Source: CAD feature listing. Evaluate the final solid. Frame: model axes, mm. A direction names the side the tool comes from. Give positions to 0.01 mm unless a question says otherwise; leave off trailing zeros. Order: outer loops, then holes, each group sorted by start corner. A loop starts at its lowest first (then second) coordinate and runs counter-clockwise, first axis right, second up. Notation, with made-up numbers: (77, 37.25) - (126, 37.25) arc R18 ccw to (126, 58.25) - close; hole circle Ø4 at (21.5, 79.25). An arc over 180 degrees is marked (long way). One line per item, written item: value. Start each with the question number.
from build123d import *

# Parameters (mm, degrees)
SKETCH1_W           = 57.15
SKETCH1_H           = 88.9
BOSS_EXTRUDE1_DEPTH = 6.35
SKETCH2_R           = 2.0193
SKETCH2_W           = 44.45
SKETCH2_H           = 19.05
CUT_EXTRUDE1_DEPTH  = 6.35
SKETCH3_W           = 6.35
SKETCH3_H           = 9.525
SKETCH3_W_2         = 9.525
SKETCH3_H_2         = 6.35
BOSS_EXTRUDE3_DEPTH = 6.35


with BuildPart() as part:
    # Sketch1 → Boss-Extrude1 (new body)
    with BuildSketch(Plane.XY):
        with Locations((28.575, -44.45)):
            Rectangle(SKETCH1_W, SKETCH1_H)
    extrude(amount=BOSS_EXTRUDE1_DEPTH)

    # Sketch2 → Cut-Extrude1 (cut)
    with BuildSketch(Plane.XY.offset(6.35)):
        with Locations((42.3926, -9.652)):
            Circle(SKETCH2_R)
        with Locations((42.3926, -38.608)):
            Circle(SKETCH2_R)
        with Locations((14.7574, -38.6842)):
            Circle(SKETCH2_R)
        with Locations((14.7574, -9.652)):
            Circle(SKETCH2_R)
        with BuildLine():
            Line((38.735, 0), (38.735, -38.1))
            ThreePointArc((38.735, -38.1), (28.575, -48.26), (18.415, -38.1))
            Line((18.415, -38.1), (18.415, 0))
            ThreePointArc((18.415, 0), (28.575, 10.16), (38.735, 0))
        make_face()
        with Locations((28.575, -73.025)):
            Rectangle(SKETCH2_W, SKETCH2_H)
    extrude(amount=-CUT_EXTRUDE1_DEPTH, mode=Mode.SUBTRACT)

    # Sketch3 → Boss-Extrude3 (add)
    with BuildSketch(Plane.XY):
        with Locations((-3.175, -14.2875)):
            Rectangle(SKETCH3_W, SKETCH3_H)
        with Locations((-3.175, -33.3375)):
            Rectangle(SKETCH3_W, SKETCH3_H)
        with Locations((-3.175, -52.3875)):
            Rectangle(SKETCH3_W, SKETCH3_H)
        with Locations((-3.175, -71.4375)):
            Rectangle(SKETCH3_W, SKETCH3_H)
        with Locations((4.7625, -92.075)):
            Rectangle(SKETCH3_W_2, SKETCH3_H_2)
        with Locations((60.325, -71.4375)):
            Rectangle(SKETCH3_W, SKETCH3_H)
        with Locations((60.325, -52.3875)):
            Rectangle(SKETCH3_W, SKETCH3_H)
        with Locations((60.325, -33.3375)):
            Rectangle(SKETCH3_W, SKETCH3_H)
        with Locations((60.325, -14.2875)):
            Rectangle(SKETCH3_W, SKETCH3_H)
        with Locations((23.8125, -92.075)):
            Rectangle(SKETCH3_W_2, SKETCH3_H_2)
        with Locations((42.8625, -92.075)):
            Rectangle(SKETCH3_W_2, SKETCH3_H_2)
    extrude(amount=BOSS_EXTRUDE3_DEPTH)


solid = part.part
1. Set-up query: faces 1 (the flat face through (60, -9.525, 3)), 2 (the flat face through (-3, -38.1, 3)), 3 (the flat face through (-3, -9.525, 3)), 4 (the flat face through (60, -38.1, 3)), 5 (the flat face through (0, -86, 3)). Return all of +Z, -Z, +X, -X, +Y, -Y with unobstructed straight access to the full face (end or side cutting, diameter ignored); none if empty.
2. Section B-B on x = 14.5. Return the cut outline in (y, z), then the cut area to 3 significant figures.
3. Ray query, L1, parallel to X at y = -15.5, z = 5.75 (3 decimals); L2, parallel to X at y = -74, z = 2.5; L3, parallel to Y at x = 28.5, z = 4. Return the intervals inside material, ascending.
4. Section A-A on y = -17. Return the cut outline in (x, z) (3 decimals).
5. Contact query for flat-ended pins moving along their axis: pin 1 Ø3 at (y, z) = (-91, 3.5) entering from -X; pin 2 Ø1.9 at (x, z) = (58.5, 4.5) entering from -Y; pin 3 Ø3 at (x, z) = (-3, 3) entering from +Y (3 decimals). Output: stop coordinate, or through.
6. Section C-C on y = -69.5. Return the cut outline in (x, z), then the cut area to 3 significant figures.
7. Section D-D on z = 4.5. Count the separate pieces of the cut face and the enclosed holes in it, then the cut area to 3 significant figures.
Data:
1. face 1: +Z, -Z, +X, +Y
1. face 2: +Z, -Z, -X
1. face 3: +Z, -Z, -X, +Y
1. face 4: +Z, -Z, +X
1. face 5: +Z, -Z, -X, -Y
2. outline: (-88.9, 0) - (-82.55, 0) - (-82.55, 6.35) - (-88.9, 6.35) - close; (-63.5, 0) - (-40.69, 0) - (-40.69, 6.35) - (-63.5, 6.35) - close; (-36.68, 0) - (-11.65, 0) - (-11.65, 6.35) - (-36.68, 6.35) - close; (-7.65, 0) - (0, 0) - (0, 6.35) - (-7.65, 6.35) - close
2. area: 393 mm2
3. L1: x = -6.35 to 18.415, 38.735 to 63.5
3. L2: x = -6.35 to 6.35, 50.8 to 63.5
3. L3: y = -95.25 to -82.55, -63.5 to -48.26
4. outline: (-6.35, 0) - (18.415, 0) - (18.415, 6.35) - (-6.35, 6.35) - close; (38.735, 0) - (63.5, 0) - (63.5, 6.35) - (38.735, 6.35) - close
5. pin 1: stops at x = 0
5. pin 2: stops at y = -76.2
5. pin 3: stops at y = -9.525
6. outline: (-6.35, 0) - (6.35, 0) - (6.35, 6.35) - (-6.35, 6.35) - close; (50.8, 0) - (63.5, 0) - (63.5, 6.35) - (50.8, 6.35) - close
6. area: 161 mm2
7. separate pieces: 1
7. enclosed holes: 5
7. area: 3,910 mm2
